Source: CAD feature listing. Evaluate the final solid. Frame: model axes, mm. Face numbers are marked on the shaded views. A direction names the side the tool comes from. Coordinates: 2 decimals unless noted, no trailing zeros. Loops run counter-clockwise (first coordinate to the right, second up) from the corner with the lowest first, then second, coordinate; pieces in that order, holes last. Notation, with made-up numbers: (53, 85.25) - (93, 85.25) arc R22 cw to (93, 118.25) - close; hole circle Ø9 at (58.5, 87). An arc over 180 degrees is marked (long way). Use CSV: the item, a comma, the result in double quotes. Start each with the question number.
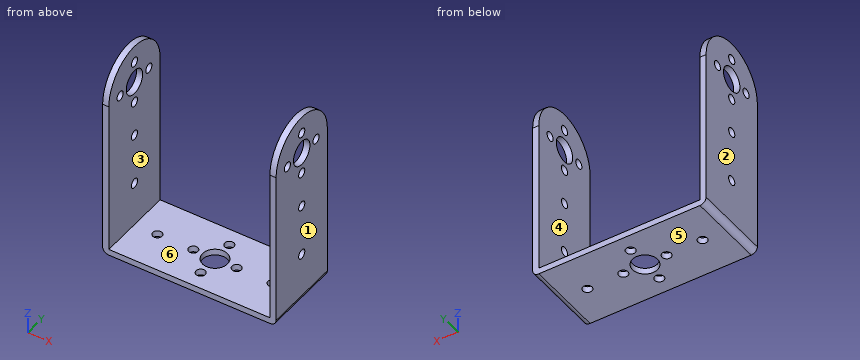
Autodesk Inventor part; units mm, degrees
ref_plane "YZ Plane" through (0, 0, 0) normal (1, 0, 0) x (0, 1, 0)
ref_plane "XZ Plane" through (0, 0, 0) normal (0, 1, 0) x (-1, 0, 0)
ref_plane "XY Plane" through (0, 0, 0) normal (0, 0, 1) x (1, 0, 0)
sketch "Sketch1" plane through (0, 0, 0) normal (0, 0, 1) x (1, 0, 0)
  line L0 (0, 0) -> (52, 0)
  line L1 (52, 0) -> (52, 25)
  line L2 (52, 25) -> (0, 25)
  line L3 (0, 25) -> (0, 0)
  circle A0 centre (26, 19.5) radius 1.5
  circle A1 centre (19, 12.5) radius 1.5
  circle A2 centre (33, 12.5) radius 1.5
  circle A3 centre (26, 5.5) radius 1.5
  circle A4 centre (7.4, 12.5) radius 1.5
  circle A5 centre (44.6, 12.5) radius 1.5
  circle A6 centre (26, 12.5) radius 4.0289
  line L4 (52, 25) -> (54, 25)
  line L5 (54, 25) -> (54, 0)
  line L6 (54, 0) -> (52, 0)
  line L7 (52, 0) -> (52, 25)
  line L8 (0, 25) -> (-2, 25)
  line L9 (-2, 25) -> (-2, 0)
  line L10 (-2, 0) -> (0, 0)
  line L11 (0, 0) -> (0, 25)
  dimension "d0" = 52
  dimension "d1" = 25
  dimension "d2" = 3
  dimension "d3" = 3
  dimension "d4" = 3
  dimension "d5" = 3
  dimension "d6" = 3
  dimension "d7" = 3
  dimension "d9" = 7.4
  dimension "d10" = 7.4
  dimension "d11" = 26
  dimension "d13" = 2
  dimension "d14" = 2
extrude "Extrusion1" add sketch "Sketch1" along normal blind 2 contours L3 L2 L1 L0
extrude "Extrusion2" add sketch "Sketch1" along normal blind 3 contours L10 L9 L8 L3 | L1 L4 L5 L6
sketch "Sketch2" plane through (0, 0, 3) normal (0, 0, 1) x (1, 0, 0)
  line L0 (54, 25) -> (-2, 25)
  line L1 (0, 0) -> (0, 25)
  line L2 (-2, 25) -> (0, 25)
  line L3 (0, 25) -> (0, 0)
  line L4 (0, 0) -> (-2, 0)
  line L5 (-2, 0) -> (-2, 25)
  line L6 (52, 25) -> (52, 0)
  line L7 (54, 0) -> (54, 25)
  line L8 (52, 25) -> (54, 25)
  line L9 (54, 25) -> (54, 0)
  line L10 (54, 0) -> (52, 0)
  line L11 (52, 0) -> (52, 25)
extrude "Extrusion3" add sketch "Sketch2" along normal blind 49
sketch "Sketch3" plane through (54, 0, 0) normal (1, 0, 0) x (0, 0, -1)
  line L0 (-52, 0) -> (-52, 25)
  line L1 (-2, 25) -> (-52, 25)
  line L2 (-2, 0) -> (-52, 0)
  arc A0 (-52, 25) -> (-52, 0) centre (-52, 12.5) ccw
  line L3 (-52, 0) -> (-52, 25)
  point P0 (0, 0)
  dimension "d22" = 12.5
extrude "Extrusion4" add sketch "Sketch3" against normal blind 2
sketch "Sketch4" plane through (-2, 0, 0) normal (-1, 0, 0) x (0, 0, 1)
  arc A0 (52, 0) -> (52, 25) centre (52, 12.5) ccw
  line L0 (2, 25) -> (52, 25)
  arc A1 (52, 0) -> (52, 25) centre (52, 12.5) ccw
  line L1 (52, 25) -> (52, 0)
  point P0 (0, 0)
extrude "Extrusion5" add sketch "Sketch4" against normal blind 2
fillet "Fillet1" radius 2 2 edges at (54, 12.5, 0) (-2, 12.5, 0)
sketch "Sketch5" plane through (-2, 12.5, 52) normal (-1, 0, 0) x (0, 0, 1)
  circle A0 centre (0, 0) radius 4
  circle A1 centre (0, 0) radius 7
  circle A2 centre (0, 7) radius 1.5
  circle A3 centre (-7, 0) radius 1.5
  circle A4 centre (0, -7) radius 1.5
  circle A5 centre (7, 0) radius 1.5
  circle A6 centre (-18.6, 0) radius 1.3978
  circle A7 centre (-35.47, 0) radius 1.5
  point P0 (-52, -12.5)
  dimension "d29" = 14
  dimension "d28" = 8
  dimension "d32" = 360
  dimension "d34" = 3
  dimension "d35" = 18.6
  dimension "d50" = 3
  dimension "d51" = 16.87
hole "Hole1" at (-2, 12.5, 52) at (-2, 12.5, 45) at (-2, 19.5, 52) at (-2, 12.5, 59) at (-2, 5.5, 52) at (-2, 12.5, 33.4) direction (1, 0, 0) diameter 3 end through all
hole "Hole2" at (-2, 12.5, 52) direction (1, 0, 0) diameter 8 end through all
hole "Hole3" at (-2, 12.5, 16.53) direction (1, 0, 0) diameter 3 end through all
properties part number "Bracket U CORTO"
(1) Ray query, line 1 (Y direction, x = 53.45, z = 52); line 2 (X direction, y = 16.25, z = 39); line 3 (Y direction, x = 33, z = 0.9). Return the intervals inside material, ascending. Write a range as [from, to].
(2) Section B-B on x = 19. Output: boundary loops of the cut face in (y, z).
(3) Section D-D on y = 5.5. Output: boundary loops of the cut face in (x, z), plus the area to 3 significant figures.
(4) Section A-A on z = 16.53. Output: boundary loops of the cut face in (x, y).
(5) Reachability of the marked faces 5 and 6 from +Z, -Z, +X, -X, +Y, -Y: full face, straight path, thin tool, end or side. Return the list, or none.
(6) Section C-C on z = 29.5. Output: boundary loops of the cut face in (x, y), plus the area to 3 significant figures.
(7) Pin query (flat end, axial travel): pin 1 Ø2 at (x, y) = (41, 13) entering from +Z; pin 2 Ø5 at (y, z) = (12.5, 33.4) entering from -X. Return the tip coordinate at first contact, or that it passes through.
(8) Draft query along X for the marked faces 1, 2, 3 and 4. Return one class per face: released by +X, released by -X, zero draft, split by the parting line, or undercut.
Solution:
1,line 1,"y = [0, 4], [7, 8.5], [16.5, 18], [21, 25]"
1,line 2,"x = [-2, 0], [52, 54]"
1,line 3,"y = [0, 11], [14, 25]"
2,outline,"(0, 0) - (11, 0) - (11, 2) - (0, 2) - close; (14, 0) - (25, 0) - (25, 2) - (14, 2) - close"
3,outline,"(-2, 2) arc R2 ccw to (0, 0) - (24.5, 0) - (24.5, 2) - (0, 2) - (0, 50.5) - (-2, 50.5) - close; (-2, 53.5) - (0, 53.5) - (0, 62.36) - (-2, 62.36) - close; (27.5, 0) - (52, 0) arc R2 ccw to (54, 2) - (54, 50.5) - (52, 50.5) - (52, 2) - (27.5, 2) - close; (52, 53.5) - (54, 53.5) - (54, 62.36) - (52, 62.36) - close"
3,area,"334 mm²"
4,outline,"(-2, 0) - (0, 0) - (0, 11) - (-2, 11) - close; (-2, 14) - (0, 14) - (0, 25) - (-2, 25) - close; (52, 0) - (54, 0) - (54, 11) - (52, 11) - close; (52, 14) - (54, 14) - (54, 25) - (52, 25) - close"
5,face 5,"-Z, +X, -X, +Y, -Y"
5,face 6,"+Z, +Y, -Y"
6,outline,"(-2, 0) - (0, 0) - (0, 25) - (-2, 25) - close; (52, 0) - (54, 0) - (54, 25) - (52, 25) - close"
6,area,"100 mm²"
7,pin 1,"stops at z = 2"
7,pin 2,"stops at x = -2"
8,face 1,"released by +X"
8,face 2,"released by -X"
8,face 3,"undercut"
8,face 4,"undercut"
